Source: CAD feature listing. Evaluate the final solid. Frame: model axes, mm. Face numbers are marked on the shaded views. Coordinates: 2 decimals unless noted, no trailing zeros. Order: outer loops, then holes, each group sorted by start corner. A loop starts at its lowest first (then second) coordinate and runs counter-clockwise, first axis right, second up. Notation, with made-up numbers: (-14.75, 1) -> (8.25, 1) arc R25 ccw to (8.25, 19) -> close; hole circle Ø8 at (66, 57). An arc over 180 degrees is marked (long way). Write each question's results on one line, items separated by ' | '. Start each with the question number.
from build123d import *

# Parameters (mm, degrees)
BOSS_EXTRUDE1_DEPTH          = 2.5
SKETCH2_W                    = 0.75
SKETCH2_H                    = 0.75
BOSS_EXTRUDE2_DEPTH          = 8.5
BOSS_EXTRUDE2_DEPTH_BACK     = 3.25
CHAMFER1_SIZE                = 0.3
REDONDEO3_R                  = 0.7
CROQUIS5_W                   = 0.748499393
CROQUIS5_H                   = 0.75
SALIENTE_EXTRUIR4_DEPTH      = 5.7
SALIENTE_EXTRUIR4_DEPTH_BACK = 5.5
CROQUIS6_W                   = 0.748499393
CROQUIS6_H                   = 0.75
SALIENTE_EXTRUIR5_DEPTH      = 0.3
SALIENTE_EXTRUIR5_TAPER      = 45
CROQUIS7_W                   = 0.748499393
CROQUIS7_H                   = 0.75
SALIENTE_EXTRUIR6_DEPTH      = 0.3
SALIENTE_EXTRUIR6_TAPER      = 45


with BuildPart() as part:
    # Sketch1 → Boss-Extrude1 (new body)
    with BuildSketch(Plane(origin=(0, 0, 0), x_dir=(-1, 0, 0), z_dir=(0, 1, 0))):
        with BuildLine():
            Line((-2, 1.27), (2, 1.27))
            Line((2, 1.27), (4.545175415, 1.27))
            Line((4.545175415, 1.27), (5.081429124, 1.27))
            Line((5.081429124, 1.27), (5.081429124, -1.27))
            Line((5.081429124, -1.27), (4.545175415, -1.27))
            Line((4.545175415, -1.27), (2, -1.27))
            Line((2, -1.27), (-2, -1.27))
            ThreePointArc((-2, -1.27), (-2.353553391, -1.123553391), (-2.5, -0.77))
            Line((-2.5, -0.77), (-2.5, 0.77))
            ThreePointArc((-2.5, 0.77), (-2.353553391, 1.123553391), (-2, 1.27))
        make_face()
    extrude(amount=BOSS_EXTRUDE1_DEPTH)

    # Sketch2 → Boss-Extrude2 (add, two sides)
    with BuildSketch(Plane(origin=(0, 0, 0), x_dir=(-1, 0, 0), z_dir=(0, 1, 0))) as boss_extrude2_sk:
        with Locations((1.27, 0)):
            Rectangle(SKETCH2_W, SKETCH2_H)
        with Locations((-1.27, 0)):
            Rectangle(SKETCH2_W, SKETCH2_H)
    extrude(amount=BOSS_EXTRUDE2_DEPTH)
    extrude(boss_extrude2_sk.sketch, amount=-BOSS_EXTRUDE2_DEPTH_BACK)

    # Chamfer1
    chamfer1_edges = [part.edges().sort_by_distance(p)[0] for p in [
        (-0.895, -3.25, 0),
        (-1.27, -3.25, 0.375),
        (-1.645, -3.25, 0),
        (-1.27, -3.25, -0.375),
        (-0.895, 8.5, 0),
        (-1.27, 8.5, -0.375),
        (-1.645, 8.5, 0),
        (-1.27, 8.5, 0.375),
        (0.895, -3.25, 0),
        (1.27, -3.25, -0.375),
        (1.645, -3.25, 0),
        (1.27, -3.25, 0.375),
        (0.895, 8.5, 0),
        (1.27, 8.5, 0.375),
        (1.645, 8.5, 0),
        (1.27, 8.5, -0.375),
    ]]
    chamfer(chamfer1_edges, length=CHAMFER1_SIZE)

    # Redondeo3
    redondeo3_edges = [part.edges().sort_by_distance(p)[0] for p in [
        (-5.081429124, 1.25, 1.27),
        (-5.081429124, 1.25, -1.27),
    ]]
    fillet(redondeo3_edges, radius=REDONDEO3_R)

    # Croquis5 → Saliente-Extruir4 (add, two sides)
    with BuildSketch(Plane(origin=(0, 2.5, 0), x_dir=(1, 0, 0), z_dir=(0, 1, 0))) as saliente_extruir4_sk:
        with Locations((-3.809249697, 0)):
            Rectangle(CROQUIS5_W, CROQUIS5_H)
    extrude(amount=SALIENTE_EXTRUIR4_DEPTH)
    extrude(saliente_extruir4_sk.sketch, amount=-SALIENTE_EXTRUIR4_DEPTH_BACK)

    # Croquis6 → Saliente-Extruir5 (add)
    with BuildSketch(Plane(origin=(0, 8.2, 0), x_dir=(1, 0, 0), z_dir=(0, 1, 0))):
        with Locations((-3.809249697, 0)):
            Rectangle(CROQUIS6_W, CROQUIS6_H)
    extrude(amount=SALIENTE_EXTRUIR5_DEPTH, taper=SALIENTE_EXTRUIR5_TAPER)

    # Croquis7 → Saliente-Extruir6 (add)
    with BuildSketch(Plane.XZ.offset(3)):
        with Locations((-3.809249697, 0)):
            Rectangle(CROQUIS7_W, CROQUIS7_H)
    extrude(amount=SALIENTE_EXTRUIR6_DEPTH, taper=SALIENTE_EXTRUIR6_TAPER)


solid = part.part
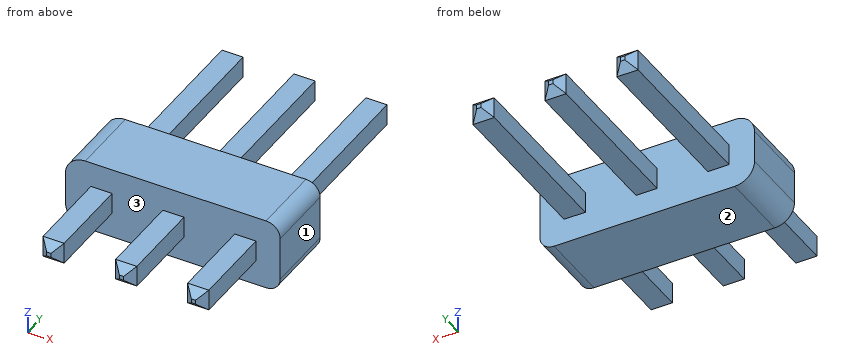
(1) Section A-A on y = 5.75. Return the cut outline in (x, z) (1 decimal), then the cut area to 3 significant figures.
(2) Line query: L1, parallel to X at y = 4, z = -0.1 (1 decimal); L2, parallel to Y at x = 1, z = 0.5; L3, parallel to Z at x = 1.25, y = -1.25 (3 decimals). Output: solid intervals per line, ascending.
(3) Section B-B on y = 1. Return the cut outline in (x, z), then the cut area to 3 significant figures.
(4) First-contact query: P1, Ø0.6, axis at y = 6.5, z = 0, coming from the +X side (3 decimals); P2, Ø0.8, axis at x = 1, y = -2, coming from the +Z side (3 decimals); P3, Ø1.5, axis at y = 7, z = 0.5, coming from the -X side. Flat tips, straight axial feed; report the tip coordinate or a pass-through.
(5) Draft query along X for the marked faces 1, 2 and 3. Return one class per face: released by +X, released by -X, zero draft, split by the parting line, or undercut.
(6) Section C-C on x = -1.5. Return the cut outline in (y, z) (3 decimals), then the cut area to 3 significant figures.
Results list:
1) outline: (-4.2, -0.4) -> (-3.4, -0.4) -> (-3.4, 0.4) -> (-4.2, 0.4) -> close; (-1.6, -0.4) -> (-0.9, -0.4) -> (-0.9, 0.4) -> (-1.6, 0.4) -> close; (0.9, -0.4) -> (1.6, -0.4) -> (1.6, 0.4) -> (0.9, 0.4) -> close | area: 1.69 mm²
2) L1: x = -4.2 to -3.4, -1.6 to -0.9, 0.9 to 1.6 | L2: y = 0 to 2.5 | L3: z = -0.375 to 0.375
3) outline: (-5.08, -0.57) arc R0.7 ccw to (-4.38, -1.27) -> (2, -1.27) arc R0.5 ccw to (2.5, -0.77) -> (2.5, 0.77) arc R0.5 ccw to (2, 1.27) -> (-4.38, 1.27) arc R0.7 ccw to (-5.08, 0.57) -> close | area: 18.9 mm²
4) P1: stops at x = 1.645 | P2: stops at z = 0.375 | P3: stops at x = -4.18
5) face 1: released by +X | face 2: zero draft | face 3: undercut
6) outline: (-3.095, -0.23) -> (-2.95, -0.375) -> (0, -0.375) -> (0, -1.27) -> (2.5, -1.27) -> (2.5, -0.375) -> (8.2, -0.375) -> (8.345, -0.23) -> (8.345, 0.23) -> (8.2, 0.375) -> (2.5, 0.375) -> (2.5, 1.27) -> (0, 1.27) -> (0, 0.375) -> (-2.95, 0.375) -> (-3.095, 0.23) -> close | area: 13.0 mm²
